from build123d import *

# Parameters (mm, degrees)
SKETCH1_R           = 3.175
BOSS_EXTRUDE1_DEPTH = 3.175


with BuildPart() as part:
    # Sketch1 → Boss-Extrude1 (new body)
    with BuildSketch(Plane.XY):
        Polygon((0, 0), (457.2, 0), (457.2, 25.4), (202.879636828, 99.242148944), (0, 25.4), align=None)
        with Locations((230.698777852, 84.552587242)):
            Circle(SKETCH1_R, mode=Mode.SUBTRACT)
        with Locations((328.269214348, 56.222922191)):
            Circle(SKETCH1_R, mode=Mode.SUBTRACT)
        with Locations((425.839650845, 27.89325714)):
            Circle(SKETCH1_R, mode=Mode.SUBTRACT)
        with Locations((31.75, 19.301847719)):
            Circle(SKETCH1_R, mode=Mode.SUBTRACT)
        with Locations((31.75, 6.35)):
            Circle(SKETCH1_R, mode=Mode.SUBTRACT)
        with Locations((158.75, 19.301847719)):
            Circle(SKETCH1_R, mode=Mode.SUBTRACT)
        with Locations((285.75, 19.301847719)):
            Circle(SKETCH1_R, mode=Mode.SUBTRACT)
        with Locations((412.75, 19.301847719)):
            Circle(SKETCH1_R, mode=Mode.SUBTRACT)
        with Locations((158.75, 6.35)):
            Circle(SKETCH1_R, mode=Mode.SUBTRACT)
        with Locations((285.75, 6.35)):
            Circle(SKETCH1_R, mode=Mode.SUBTRACT)
        with Locations((412.75, 6.35)):
            Circle(SKETCH1_R, mode=Mode.SUBTRACT)
    extrude(amount=BOSS_EXTRUDE1_DEPTH)


solid = part.part
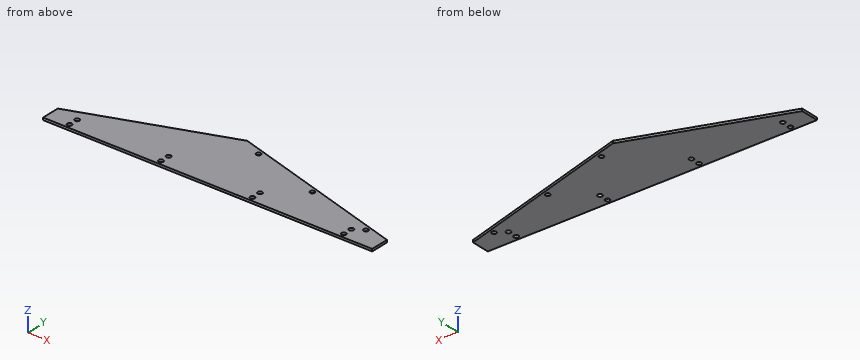
CAD build for the part. Positions are in the model's coordinates, mm. Give positions to 0.01 mm unless a question says otherwise; leave off trailing zeros. Loops run counter-clockwise (first coordinate to the right, second up) from the corner with the lowest first, then second, coordinate; pieces in that order, holes last. Notation, with made-up numbers: M -33,-3.75 L 11,-3.75 A15 ccw 11,0.25 Z; hole C 65.5,-30 d8. An arc over 180 degrees is marked long. Answer in a Markdown table with one row per item. Add a question column.
Item 1: Band-saw the part on C-C on x = 260. Give the cut face in (y, z) (3 decimals).
Item 2: Probe probe 1 along Y at (x, z) = (158.75, 1.05) (3 decimals); probe 2 along Y at (x, z) = (285.75, 2.15) (3 decimals); probe 3 along Y at (x, z) = (178, 2). List the from-to ranges inside material, lowest first.
Item 3: Band-saw the part on B-B on y = 37.5. Give the cut face in (x, z) (3 decimals).
Item 4: Band-saw the part on A-A on z = 2.5. Give the number of separate pieces and of enclosed holes in the cut face, then the cut area to 3 significant figures.
Item 5: Drop flat-ended pins along their axis: P1, Ø1, axis at x = 173, z = 1.5, coming from the +Y side; P2, Ø5.5, axis at x = 158.75, y = 6.35, coming from the -Z side. Give the stop position or say it passes through.
Reply:
| question | item | result |
|---|---|---|
| 1 | outline | M 0,0 L 82.657,0 L 82.657,3.175 L 0,3.175 Z |
| 2 | probe 1 | y = 0 to 3.175, 9.525 to 16.127, 22.477 to 83.18 |
| 2 | probe 2 | y = 0 to 3.175, 9.525 to 16.127, 22.477 to 75.181 |
| 2 | probe 3 | y = 0 to 90.19 |
| 3 | outline | M 33.244,0 L 415.526,0 L 415.526,3.175 L 33.244,3.175 Z |
| 4 | separate pieces | 1 |
| 4 | enclosed holes | 11 |
| 4 | area | 28,100 mm^2 |
| 5 | P1 | stops at y = 88.55 |
| 5 | P2 | passes through |
